```python
from build123d import *

# Parameters (mm, degrees)
F0_W     = 135
F0_H     = 135
F1_DEPTH = 4
F2_R     = 1
F4_DEPTH = 6
F5_R     = 1


with BuildPart() as f1:
    # F0 (on Top) → F1 (new body)
    with BuildSketch(Plane.XY):
        with Locations((67.5, 67.5)):
            Rectangle(F0_W, F0_H)
    extrude(amount=F1_DEPTH)

    # F2
    f2_edges = [f1.edges().sort_by_distance(p)[0] for p in [
        (0, 67.5, 4),
        (67.5, 0, 4),
        (135, 67.5, 4),
        (67.5, 135, 4),
        (0, 67.5, 0),
        (67.5, 0, 0),
        (135, 67.5, 0),
        (67.5, 135, 0),
        (135, 0, 2),
        (0, 0, 2),
        (135, 135, 2),
        (0, 135, 2),
    ]]
    fillet(f2_edges, radius=F2_R)

    # F3 (on face) → F4 (join)
    with BuildSketch(Plane.XY.offset(4)):
        Polygon((22.5, 102.839746), (30, 107.169873), (30, 115.830127), (22.5, 120.160254), (15, 115.830127), (15, 107.169873), align=None)
        Polygon((120, 115.830127), (112.5, 120.160254), (105, 115.830127), (105, 107.169873), (112.5, 102.839746), (120, 107.169873), align=None)
        Polygon((30, 19.169873), (30, 27.830127), (22.5, 32.160254), (15, 27.830127), (15, 19.169873), (22.5, 14.839746), align=None)
        Polygon((105, 19.169873), (112.5, 14.839746), (120, 19.169873), (120, 27.830127), (112.5, 32.160254), (105, 27.830127), align=None)
    extrude(amount=F4_DEPTH)

    # F5
    f5_edges = [f1.edges().sort_by_distance(p)[0] for p in [
        (26.25, 105.004809, 10),
        (30, 111.5, 10),
        (26.25, 117.995191, 10),
        (18.75, 117.995191, 10),
        (15, 111.5, 10),
        (18.75, 105.004809, 10),
        (116.25, 105.004809, 10),
        (120, 111.5, 10),
        (116.25, 117.995191, 10),
        (108.75, 117.995191, 10),
        (105, 111.5, 10),
        (108.75, 105.004809, 10),
        (108.75, 29.995191, 10),
        (105, 23.5, 10),
        (108.75, 17.004809, 10),
        (116.25, 17.004809, 10),
        (120, 23.5, 10),
        (116.25, 29.995191, 10),
        (26.25, 17.004809, 10),
        (30, 23.5, 10),
        (26.25, 29.995191, 10),
        (18.75, 29.995191, 10),
        (15, 23.5, 10),
        (18.75, 17.004809, 10),
    ]]
    fillet(f5_edges, radius=F5_R)


solid = f1.part
```
Can you work these out from the model? Positions are in its coordinate system, mm. A direction names the side the tool comes from. Give positions to 0.01 mm unless a question says otherwise; leave off trailing zeros. Loops run counter-clockwise (first coordinate to the right, second up) from the corner with the lowest first, then second, coordinate; pieces in that order, holes last. Notation, with made-up numbers: M 86,-36 L 113,-36 A16 cw 113,-12 Z; hole C 45.25,4.5 d11. An arc over 180 degrees is marked long. Use one line per item in the form item = value. Start each with the question number.
(1) Please list where these lines run through material, in increasing order: line 1 (Z direction, x = 11, y = 95); line 2 (Y direction, x = 27, z = 7.25); line 3 (X direction, y = 17.5, z = 9.25).
(2) On a 3-axis mill with a long thin cutter (end or side, diameter ignored), from which of +Z, -Z, +X, -X, +Y, -Y can I reach the whole of each face in a straight line? I mean faces 4 (the flat face through (108.802, 118.026, 6.465)), 5 (the flat face through (30, 23, 6)), 6 (the cylindrical face through (26.16, 17.28, 9.7)), 7 (the flat face through (18.698, 105.035, 6.465)), 8 (the flat face through (120, 23, 6)). Say none if no direction works.
(3) I'm going to push flat-ended pins straight in: P1, Ø6, axis at x = 101, y = 35.5, coming from the +Z side; P2, Ø4, axis at y = 22, z = 7, coming from the +X side; P3, Ø1.5, axis at y = 23.5, z = 6, coming from the -X side; P4, Ø6, axis at y = 38, z = 8.5, coming from the +X side. Where does each tip first touch, or does it pass through?
(4) I want a section at C-C, the plane x = 103. Write out the boundary of the cut face in (y, z).
(5) I want a section at A-A, the plane z = 6.25. Write out the boundary of the cut face in (x, y), and give its area (3 significant figures).
(6) Thinking about a two-plate mould opening in Y: for faces 1 (the flat face through (105, 112, 6)), 2 (the flat face through (18.698, 17.035, 6.465)), 3 (the cylindrical face through (18.95, 105.22, 9.7)), which applies, released by +Y, released by -Y, zero draft, split by the parting line, or undercut?
(7) I want a section at B-B, the plane y = 25.5. Write out the boundary of the cut face in (x, z), and give its area (3 significant figures).
Worked out:
q1.line_1 = 0 to 4
q1.line_2 = 17.44 to 29.56, 105.44 to 117.56
q1.line_3 = 17.96 to 27.04, 107.96 to 117.04
q2.face_4 = +Z, +Y
q2.face_5 = +Z, +Y, -Y
q2.face_6 = +Z, -Y
q2.face_7 = +Z, -X
q2.face_8 = +Z, +X, +Y, -Y
q3.P1 = 4
q3.P2 = 120
q3.P3 = 15
q3.P4 = through
q4.outline = M 0,1 A1 ccw 1,0 L 134,0 A1 ccw 135,1 L 135,3 A1 ccw 134,4 L 1,4 A1 ccw 0,3 Z
q5.outline = M 15,19.17 L 22.5,14.84 L 30,19.17 L 30,27.83 L 22.5,32.16 L 15,27.83 Z; M 15,107.17 L 22.5,102.84 L 30,107.17 L 30,115.83 L 22.5,120.16 L 15,115.83 Z; M 105,19.17 L 112.5,14.84 L 120,19.17 L 120,27.83 L 112.5,32.16 L 105,27.83 Z; M 105,107.17 L 112.5,102.84 L 120,107.17 L 120,115.83 L 112.5,120.16 L 105,115.83 Z
q5.area = 779 mm²
q6.face_1 = zero draft
q6.face_2 = released by -Y
q6.face_3 = undercut
q7.outline = M 0,1 A1 ccw 1,0 L 134,0 A1 ccw 135,1 L 135,3 A1 ccw 134,4 L 120,4 L 120,9 A1 ccw 119,10 L 106,10 A1 ccw 105,9 L 105,4 L 30,4 L 30,9 A1 ccw 29,10 L 16,10 A1 ccw 15,9 L 15,4 L 1,4 A1 ccw 0,3 Z
q7.area = 718 mm²
